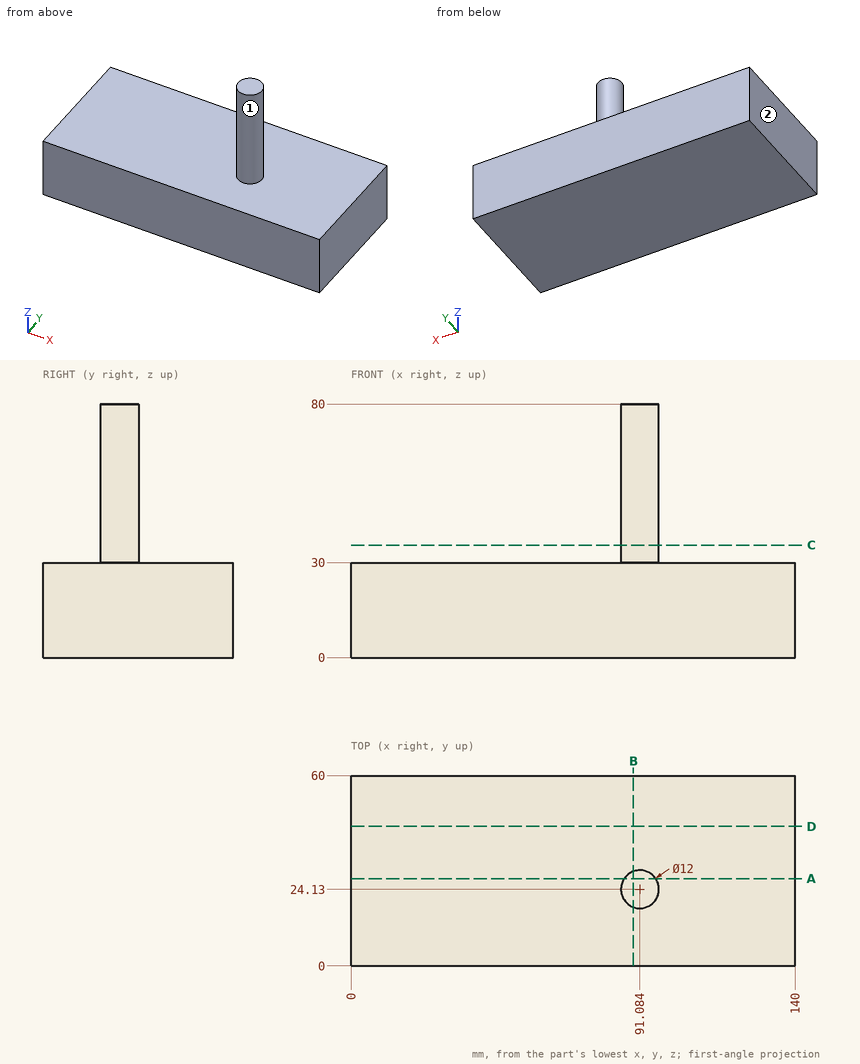
Check sheet for the drawn part. Datum: minimum x, y, z corner. Units: mm. A direction names the side the tool comes from. Give positions to 0.01 mm unless a question says otherwise; leave off trailing zeros. Order: outer loops, then holes, each group sorted by start corner. A loop starts at its lowest first (then second) coordinate and runs counter-clockwise, first axis right, second up. Notation, with made-up numbers: (74.5, 43.5) -> (124.5, 43.5) arc R18 ccw to (124.5, 50.5) -> close; hole circle Ø8 at (67.25, 76). An arc over 180 degrees is marked (long way). Return JSON: item names as keys, results as strings.
1. Go/stop test with flat-tipped pins: P1, Ø6, axis at y = 27, z = 28, coming from the -X side; P2, Ø10, axis at y = 10.5, z = 61.5, coming from the -X side; P3, Ø18, axis at x = 81, y = 40, coming from the +Z side. Record where each tip stops, or that it passes through.
From the geometry:
{"P1": "x = 0", "P2": "through", "P3": "z = 30"}
2. Set-up check for the marked faces 1 and 2: record each of +Z, -Z, +X, -X, +Y, -Y from which the full face is reachable in a straight line by a thin tool's end or side.
From the geometry:
{"face 1": "+Z", "face 2": "+Z, -Z, -X, +Y, -Y"}
3. Cross-section at C-C, the plane z = 35.5. Record the cut outline in (x, y), plus the area to 3 significant figures.
From the geometry:
{"outline": "circle Ø12 at (91.08, 24.13)", "area": "113 mm^2"}
4. Cross-section at B-B, the plane x = 89. Record the cut outline in (y, z).
From the geometry:
{"outline": "(0, 0) -> (60, 0) -> (60, 30) -> (29.76, 30) -> (29.76, 80) -> (18.5, 80) -> (18.5, 30) -> (0, 30) -> close"}
5. Material ranges on probe 1 along Z at (x, y) = (11, 31); probe 2 along Y at (x, z) = (89, 59), recorded low to high. Write a range as [from, to].
From the geometry:
{"probe 1": "[0, 30]", "probe 2": "[18.5, 29.76]"}
6. Cross-section at D-D, the plane y = 44. Record the cut outline in (x, z), plus the area to 3 significant figures.
From the geometry:
{"outline": "(0, 0) -> (140, 0) -> (140, 30) -> (0, 30) -> close", "area": "4,200 mm^2"}
7. Cross-section at A-A, the plane y = 27.5. Record the cut outline in (x, z).
From the geometry:
{"outline": "(0, 0) -> (140, 0) -> (140, 30) -> (96.05, 30) -> (96.05, 80) -> (86.12, 80) -> (86.12, 30) -> (0, 30) -> close"}
